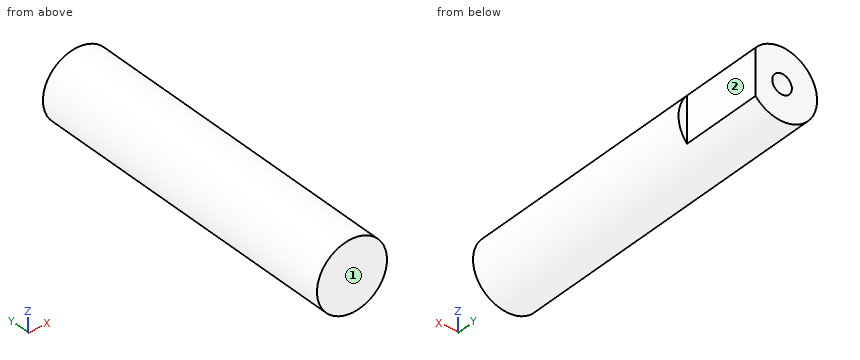
from build123d import *

# Parameters (mm, degrees)
F0_R     = 12.5
F1_DEPTH = 120
F3_D     = 7
F3_DEPTH = 40
F3_TIP   = 2.1030121666
F5_W     = 30
F5_H     = 30.6473458186
F6_DEPTH = 3


with BuildPart() as f1:
    # F0 (on Front) → F1 (new body)
    with BuildSketch(Plane.XZ):
        Circle(F0_R)
    extrude(amount=F1_DEPTH)

    # F3
    with Locations(Plane(origin=(0, 0, 0), x_dir=(-1, 0, 0), z_dir=(0, 1, 0))):
        with Locations((0, 0)):
            Hole(F3_D / 2, depth=F3_DEPTH)
            with Locations((0, 0, -(F3_DEPTH + F3_TIP / 2))):  # 118° drill point
                Cone(0, F3_D / 2, F3_TIP, mode=Mode.SUBTRACT)

    # F5 (on offset) → F6 (cut)
    with BuildSketch(Plane.YZ.offset(12.5)):
        with Locations((-15, -0.2489075996)):
            Rectangle(F5_W, F5_H)
    extrude(amount=-F6_DEPTH, mode=Mode.SUBTRACT)


solid = f1.part
Read the model definition and answer for the solid it produces. Units are mm, in the model's axes. Face numbers are marked on the shaded views. A direction names the side the tool comes from. Coordinates: 2 decimals unless noted, no trailing zeros. Loops run counter-clockwise (first coordinate to the right, second up) from the corner with the lowest first, then second, coordinate; pieces in that order, holes last. Notation, with made-up numbers: (81, -35) -> (128, -35) arc R7 ccw to (128, -23) -> close; hole circle Ø4 at (12, 68). An arc over 180 degrees is marked (long way). Answer in a Markdown table with one row per item.
Item 1: A cutting plane is placed at D-D on z = -7. Determine the outline of the cut face in (x, y).
Returned:
| item | result |
|---|---|
| outline | (-10.36, -120) -> (10.36, -120) -> (10.36, -30) -> (9.5, -30) -> (9.5, 0) -> (-10.36, 0) -> close |
Item 2: A cutting plane is placed at B-B on z = 9.5. Determine the outline of the cut face in (x, y), plus the area to 3 significant figures.
Returned:
| item | result |
|---|---|
| outline | (-8.12, -120) -> (8.12, -120) -> (8.12, 0) -> (-8.12, 0) -> close |
| area | 1,950 mm^2 |
Item 3: Straight lines are drawn through the part: line 1 along X through (y, z) = (-16, 0); line 2 along Z through (x, y) = (0, -23); line 3 along Z through (x, y) = (-4, -25.5). For each, find the intervals that lie inside material, in ascending order. Write a range as [from, to].
Returned:
| item | result |
|---|---|
| line 1 | x = [-12.5, -3.5], [3.5, 9.5] |
| line 2 | z = [-12.5, -3.5], [3.5, 12.5] |
| line 3 | z = [-11.84, 11.84] |
Item 4: A cutting plane is placed at A-A on y = -19. Determine the outline of the cut face in (x, z).
Returned:
| item | result |
|---|---|
| outline | (9.5, -8.12) -> (9.5, 8.12) arc R12.5 ccw (long way) to start; hole circle Ø7 at (0, 0) |
Item 5: For the marked faces 1 and 2, determine the directions among +Z, -Z, +X, -X, +Y, -Y from which every point of the face is accessible in a straight line to the end or side of a thin tool.
Returned:
| item | result |
|---|---|
| face 1 | +Z, -Z, +X, -X, -Y |
| face 2 | +Z, -Z, +X, +Y |
Item 6: Each of these flat-tipped pins is pushed along its axis until it touches: P1, Ø4, axis at x = 9, y = -72.5, coming from the -Z side; P2, Ø2.5, axis at x = 11.5, z = -1, coming from the +Y side; P3, Ø1, axis at y = -95.5, z = -5.5, coming from the -X side. Where does it stop, or does it pass through?
Returned:
| item | result |
|---|---|
| P1 | stops at z = -10.36 |
| P2 | stops at y = -30 |
| P3 | stops at x = -11.46 |
Item 7: A cutting plane is placed at C-C on x = 5.5. Determine the outline of the cut face in (y, z), plus the area to 3 significant figures.
Returned:
| item | result |
|---|---|
| outline | (-120, -11.22) -> (0, -11.22) -> (0, 11.22) -> (-120, 11.22) -> close |
| area | 2,690 mm^2 |
